```python
from build123d import *

# Parameters (mm, degrees)
SKETCH1_W               = 60
SKETCH1_H               = 53
BOSS_EXTRUDE1_DEPTH     = 2
SKETCH3_W               = 56
SKETCH3_H               = 12
BOSS_EXTRUDE3_DEPTH     = 10
SKETCH2_W               = 56
SKETCH2_H               = 5
BOSS_EXTRUDE2_DEPTH     = 8
CUT_EXTRUDE1_DEPTH      = 10.1
CUT_EXTRUDE1_DEPTH_BACK = 10.1
CUT_EXTRUDE2_DEPTH      = 10.1
CUT_EXTRUDE2_DEPTH_BACK = 10.1
SKETCH6_W               = 13
SKETCH6_H               = 4.05
CUT_EXTRUDE3_DEPTH      = 6
SKETCH7_R               = 1.9
BOSS_EXTRUDE4_DEPTH     = 3
BOSS_EXTRUDE4_TAPER     = 10
FILLET2_R               = 0.4
CUT_EXTRUDE4_REACH      = 53
SKETCH9_W               = 4.1
SKETCH9_H               = 1.7
CUT_EXTRUDE5_DEPTH      = 4


with BuildPart() as part:
    # Sketch1 → Boss-Extrude1 (new body)
    with BuildSketch(Plane(origin=(0, 0, 0), x_dir=(1, 0, 0), z_dir=(0, 1, 0))):
        with Locations((30, 26.5)):
            Rectangle(SKETCH1_W, SKETCH1_H)
    extrude(amount=BOSS_EXTRUDE1_DEPTH)

    # Sketch3 → Boss-Extrude3 (add)
    with BuildSketch(Plane(origin=(0, 0, 0), x_dir=(1, 0, 0), z_dir=(0, 1, 0))):
        with Locations((30, 45)):
            Rectangle(SKETCH3_W, SKETCH3_H)
    extrude(amount=BOSS_EXTRUDE3_DEPTH)

    # Sketch2 → Boss-Extrude2 (add)
    with BuildSketch(Plane(origin=(0, 0, 0), x_dir=(1, 0, 0), z_dir=(0, 1, 0))):
        with Locations((30, 6.5)):
            Rectangle(SKETCH2_W, SKETCH2_H)
    extrude(amount=BOSS_EXTRUDE2_DEPTH)

    # Sketch4 → Cut-Extrude1 (cut, two sides)
    with BuildSketch(Plane.ZY.offset(-15)) as cut_extrude1_sk:
        with BuildLine():
            Line((-40.95, 10), (-49.05, 10))
            ThreePointArc((-49.05, 10), (-45, 5.95), (-40.95, 10))
        make_face()
    extrude(amount=CUT_EXTRUDE1_DEPTH, mode=Mode.SUBTRACT)
    extrude(cut_extrude1_sk.sketch, amount=-CUT_EXTRUDE1_DEPTH_BACK, mode=Mode.SUBTRACT)

    # Sketch5 → Cut-Extrude2 (cut, two sides)
    with BuildSketch(Plane(origin=(45, 0, 0), x_dir=(0, 0, -1), z_dir=(1, 0, 0))) as cut_extrude2_sk:
        with BuildLine():
            Line((40.95, 10), (49.05, 10))
            ThreePointArc((49.05, 10), (45, 5.95), (40.95, 10))
        make_face()
    extrude(amount=CUT_EXTRUDE2_DEPTH, mode=Mode.SUBTRACT)
    extrude(cut_extrude2_sk.sketch, amount=-CUT_EXTRUDE2_DEPTH_BACK, mode=Mode.SUBTRACT)

    # Sketch6 → Cut-Extrude3 (cut)
    with BuildSketch(Plane.XY.offset(-39)):
        with Locations((15, 7.975)):
            Rectangle(SKETCH6_W, SKETCH6_H)
        with Locations((45, 7.975)):
            Rectangle(SKETCH6_W, SKETCH6_H)
    extrude(amount=-CUT_EXTRUDE3_DEPTH, mode=Mode.SUBTRACT)

    # Sketch7 → Boss-Extrude4 (add)
    with BuildSketch(Plane(origin=(0, 2, 0), x_dir=(1, 0, 0), z_dir=(0, 1, 0))):
        with Locations((15, 21.2)):
            Circle(SKETCH7_R)
        with Locations((45, 21.2)):
            Circle(SKETCH7_R)
    extrude(amount=BOSS_EXTRUDE4_DEPTH, taper=BOSS_EXTRUDE4_TAPER)

    # Fillet2
    fillet2_edges = [part.edges().sort_by_distance(p)[0] for p in [
        (58, 6, -51),
        (2, 6, -51),
        (2, 6, -39),
        (58, 6, -39),
        (2, 5, -4),
        (58, 5, -4),
        (58, 5, -9),
        (2, 5, -9),
        (0, 1, 0),
        (0, 1, -53),
        (60, 1, -53),
        (60, 1, 0),
        (8.5, 7.975, -39),
        (21.5, 7.975, -39),
        (38.5, 7.975, -39),
        (51.5, 7.975, -39),
    ]]
    fillet(fillet2_edges, radius=FILLET2_R)

    # Sketch8 → Cut-Extrude4 (cut, up to next)
    with BuildSketch(Plane(origin=(0, 0, -51), x_dir=(-1, 0, 0), z_dir=(0, 0, -1)), mode=Mode.PRIVATE) as cut_extrude4_sk1:
        Polygon((-30, 6), (-31.865230633, 2), (-28.134769367, 2), align=None)
    cut_extrude4_tool1 = extrude(cut_extrude4_sk1.sketch, amount=-CUT_EXTRUDE4_REACH, mode=Mode.PRIVATE) & part.part
    add(cut_extrude4_tool1.solids().sort_by_distance((30, 3.333333, -51))[0], mode=Mode.SUBTRACT)

    # Sketch9 → Cut-Extrude5 (cut)
    with BuildSketch(Plane(origin=(0, 8, 0), x_dir=(1, 0, 0), z_dir=(0, 1, 0))):
        with Locations((15, 8.15)):
            Rectangle(SKETCH9_W, SKETCH9_H)
        with Locations((45, 8.15)):
            Rectangle(SKETCH9_W, SKETCH9_H)
    extrude(amount=-CUT_EXTRUDE5_DEPTH, mode=Mode.SUBTRACT)


solid = part.part
```
Verification items for the finished model (mm, model axes). A direction names the side the tool comes from. Coordinates: 2 decimals unless noted, no trailing zeros. Write each loop counter-clockwise with the first axis right and the second up, starting at its lowest first coordinate (ties: lowest second). Pieces come first, ordered by that corner, then holes. Notation, with made-up numbers: M 51.25,81 L 80.25,81 A30 cw 80.25,119 Z; hole C 80,-5 d6. An arc over 180 degrees is marked long. Answer as a JSON object with one key per item and string values. Group by question number.
(1) Cross-section at A-A, the plane x = 45. Record the cut outline in (y, z).
(2) Cross-section at C-C, the plane x = 12. Record the cut outline in (y, z), and give its area (3 significant figures).
(3) Material ranges on line 1 (X direction, y = 7.5, z = -43); line 2 (Z direction, x = 5, y = 9.75); line 3 (Z direction, x = 19.5, y = 5), recorded low to high.
(4) Cross-section at B-B, the plane z = -42. Record the cut outline in (x, y), and give its area (3 significant figures).
(5) Gauge pin test, flat ends, axial feed: pin 1 (4 mm diameter, centred on y = 3, z = -32, fed in from -X); pin 2 (3 mm diameter, centred on y = 8, z = -46, fed in from -X); pin 3 (2 mm diameter, centred on x = 45, y = 5, fed in from -Z); pin 4 (1.4 mm diameter, centred on y = 5.5, z = -8, fed in from +X). Record the tip position at first contact, or that the pin passes through.
(6) Release check for a two-part mould opening along Z. For faces 1 (the face through (30, 1, -53)), 2 (the face through (15, 5, -21)), 3 (the face through (17.05, 6, -8)), 4 (the face through (58, 5, -6)) record: +Z half, -Z half, draft (parallel to the pull), parting line (faces both ways), or undercut.
(7) Tool access check on faces 5 (the face through (58, 6, -45)), 6 (the face through (34.9, 8, -45)), 7 (the face through (30, 5, -4)). Record the directions out of +Z, -Z, +X, -X, +Y, -Y that give a thin tool (end or side, any length) a straight path to the whole face; none if there is none.
Reply:
{
 "1": {"outline": "M 0,-53 L 2,-53 L 2,-51 L 10,-51 L 10,-49.05 A4.05 cw 5.95,-45 L 5.95,-39 L 2,-39 L 2,-23.1 L 5,-22.57 L 5,-19.83 L 2,-19.3 L 2,-9 L 4,-9 L 4,-7.3 L 8,-7.3 L 8,-4 L 2,-4 L 2,0 L 0,0 Z"},
 "2": {"outline": "M 0,-53 L 2,-53 L 2,-51 L 10,-51 L 10,-49.05 A4.05 cw 5.95,-45 L 5.95,-39 L 2,-39 L 2,-9 L 8,-9 L 8,-4 L 2,-4 L 2,0 L 0,0 Z", "area": "195 mm²"},
 "3": {"line 1": "2 to 4.9, 25.1 to 34.9, 55.1 to 58", "line 2": "-51 to -49.04, -40.96 to -39", "line 3": "-51 to -39, -9 to -4"},
 "4": {"outline": "M 0,0 L 60,0 L 60,2 L 58,2 L 58,10 L 55.1,10 L 55.1,7.28 L 51.5,7.28 L 51.5,5.95 L 38.5,5.95 L 38.5,7.28 L 34.9,7.28 L 34.9,10 L 25.1,10 L 25.1,7.28 L 21.5,7.28 L 21.5,5.95 L 8.5,5.95 L 8.5,7.28 L 4.9,7.28 L 4.9,10 L 2,10 L 2,2 L 0,2 Z; hole M 28.13,2 L 31.87,2 L 30,6 Z", "area": "416 mm²"},
 "5": {"pin 1": "x = 0", "pin 2": "x = 2", "pin 3": "z = -51", "pin 4": "x = 58"},
 "6": {"face 1": "-Z half", "face 2": "undercut", "face 3": "undercut", "face 4": "draft"},
 "7": {"face 5": "+Z, -Z, +X, +Y", "face 6": "+Y", "face 7": "+Z, +X, -X, +Y"}
}
